Geometry: final body of the model. Coordinates: model frame, mm. Round coordinates to 2 decimals unless told otherwise and drop trailing zeros. Loops run counter-clockwise (first coordinate to the right, second up) from the corner with the lowest first, then second, coordinate; pieces in that order, holes last. Notation, with made-up numbers: (36, -30) - (66, -30) arc R21 cw to (66, 8) - close; hole circle Ø9 at (-34, -24). An arc over 180 degrees is marked (long way). Answer as CSV lines item,"result".
from build123d import *

# Parameters (mm, degrees)
SKETCH1_W                              = 25.4
SKETCH1_H                              = 25.4
SKETCH1_W_2                            = 24.2824
SKETCH1_H_2                            = 24.2824
AL_TUBE_SQUARE_1_SQ_X_022_WALL_3_DEPTH = 1300
CROQUIS3_R                             = 6.35
CORTAR_EXTRUIR1_DEPTH                  = 1301.310136083


with BuildPart() as part:
    # Sketch1 → Al tube (square) 1 SQ X .022 WALL(3) (new body)
    with BuildSketch(Plane.YZ):
        Rectangle(SKETCH1_W, SKETCH1_H)
        Rectangle(SKETCH1_W_2, SKETCH1_H_2, mode=Mode.SUBTRACT)
    extrude(amount=AL_TUBE_SQUARE_1_SQ_X_022_WALL_3_DEPTH)

    # Croquis3 → Cortar-Extruir1 (cut, through all)
    with BuildSketch(Plane.XY.offset(12.7)):
        with Locations((1287.3, 0)):
            Circle(CROQUIS3_R)
        with Locations((900, 0)):
            Circle(CROQUIS3_R)
        with Locations((12.7, 0)):
            Circle(CROQUIS3_R)
    extrude(amount=-CORTAR_EXTRUIR1_DEPTH, mode=Mode.SUBTRACT)


solid = part.part
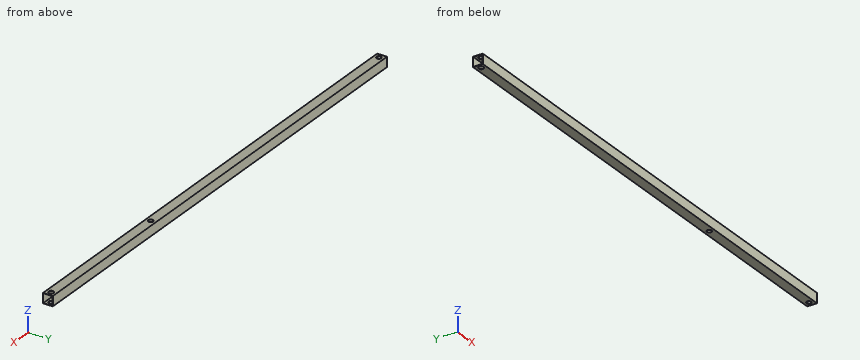
(1) Section B-B (y = 0). Give the number of separate pieces and of enclosed holes in the cut face, and give its area (3 significant figures).
Findings below:
separate pieces,"8"
enclosed holes,"0"
area,"1,410 mm2"
(2) Section C-C (z = -4.5). Output: boundary loops of the cut face in (x, y).
Findings below:
outline,"(0, -12.7) - (1300, -12.7) - (1300, -12.14) - (0, -12.14) - close; (0, 12.14) - (1300, 12.14) - (1300, 12.7) - (0, 12.7) - close"
(3) Material intervals for line 1 along Y through (x, z) = (313, 10.25); line 2 along Y through (x, z) = (12.7, 12.55), sorted ascending.
Findings below:
line 1,"-12.7 to -12.14, 12.14 to 12.7"
line 2,"-12.7 to -6.35, 6.35 to 12.7"
(4) Section A-A (x = 472). Output: boundary loops of the cut face in (y, z).
Findings below:
outline,"(-12.7, -12.7) - (12.7, -12.7) - (12.7, 12.7) - (-12.7, 12.7) - close; hole (-12.14, -12.14) - (12.14, -12.14) - (12.14, 12.14) - (-12.14, 12.14) - close"
(5) Pin query (flat end, axial travel): P1, Ø7.5, axis at x = 12.7, y = 0, coming from the +Z side. Return the tip coordinate at first contact, or that it passes through.
Findings below:
P1,"through"
